Source: CAD feature listing. Evaluate the final solid. Frame: model axes, mm. Round coordinates to 2 decimals unless told otherwise and drop trailing zeros. Write each loop counter-clockwise with the first axis right and the second up, starting at its lowest first coordinate (ties: lowest second). Pieces come first, ordered by that corner, then holes. Notation, with made-up numbers: M 85.5,-3 L 130.5,-3 A22 ccw 130.5,24 Z; hole C 62.25,16 d11. An arc over 180 degrees is marked long. Answer in a Markdown table with one row per item.
from build123d import *

# Parameters (mm, degrees)
F1_DEPTH = 19.05
F2_R     = 76.2
F3_W     = 88.9
F3_H     = 38.1
F4_DEPTH = 38.1
F6_DEPTH = 38.101


with BuildPart() as f1:
    # F0 (on Front) → F1 (new body, symmetric)
    with BuildSketch(Plane.XZ):
        Polygon((-44.45, 0), (-19.05, 0), (19.05, 0), (44.45, 0), (330.2, -433.689813), (381, -433.689813), (117.024645, 76.2), (381, 290.210187), (292.1, 290.210187), (44.45, 152.4), (0, 152.4), (-44.45, 152.4), (-292.1, 290.210187), (-381, 290.210187), (-117.024645, 76.2), (-381, -433.689813), (-330.2, -433.689813), align=None)
    extrude(amount=F1_DEPTH, both=True)

    # F2
    f2_edges = [f1.edges().sort_by_distance(p)[0] for p in [
        (117.024645, 0, 76.2),
        (-44.45, 0, 152.4),
        (44.45, 0, 152.4),
        (-117.024645, 0, 76.2),
        (-44.45, 0, 0),
        (44.45, 0, 0),
    ]]
    fillet(f2_edges, radius=F2_R)

    # F3 (on face) → F4 (join)
    with BuildSketch(Plane.XY.offset(290.210187)):
        with Locations((-336.55, 0)):
            Rectangle(F3_W, F3_H)
        with Locations((336.55, 0)):
            Rectangle(F3_W, F3_H)
    extrude(amount=F4_DEPTH)

    # F5 (on face) → F6 (cut, through all)
    with BuildSketch(Plane.XZ.offset(19.05)):
        with BuildLine():
            Line((-19.05, 76.2), (-19.05, -1.623687))
            ThreePointArc((-19.05, -1.623687), (-11.268752, -0.407009), (-3.403482, 0))
            Line((-3.403482, 0), (3.403482, 0))
            ThreePointArc((3.403482, 0), (11.268752, -0.407009), (19.05, -1.623687))
            Line((19.05, -1.623687), (19.05, 76.2))
            Line((19.05, 76.2), (-19.05, 76.2))
        make_face()
        with BuildLine():
            Line((-19.05, -1.623687), (-19.05, -12.7))
            Line((-19.05, -12.7), (19.05, -12.7))
            Line((19.05, -12.7), (19.05, -1.623687))
            ThreePointArc((19.05, -1.623687), (11.268752, -0.407009), (3.403482, 0))
            Line((3.403482, 0), (-3.403482, 0))
            ThreePointArc((-3.403482, 0), (-11.268752, -0.407009), (-19.05, -1.623687))
        make_face()
    extrude(amount=-F6_DEPTH, mode=Mode.SUBTRACT)


solid = f1.part
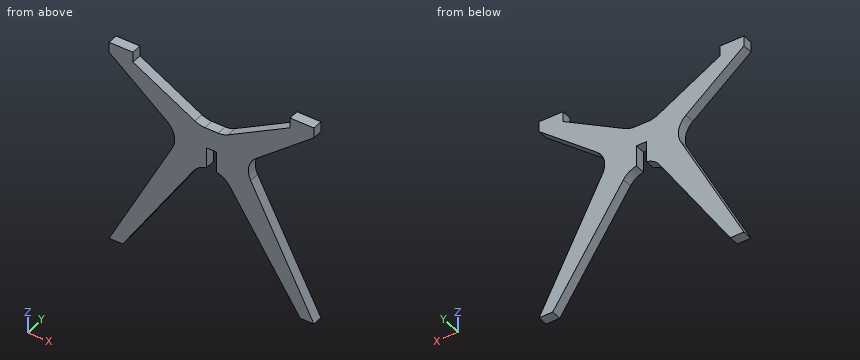
Q1. Contact query for flat-ended pins moving along their axis: pin 1 Ø19 at (y, z) = (9.5, 46) entering from +X; pin 2 Ø3 at (x, y) = (20.5, -11) entering from +Z; pin 3 Ø3 at (x, y) = (-133, 7) entering from +Z. Output: stop coordinate, or through.
Solutions:
| item | result |
|---|---|
| pin 1 | stops at x = 139.6 |
| pin 2 | stops at z = 152.4 |
| pin 3 | stops at z = 202.51 |
Q2. Section D-D (x = -86.5). Return loops of the section in (y, z).
Solutions:
| item | result |
|---|---|
| outline | M -19.05,-63.82 L 19.05,-63.82 L 19.05,175.8 L -19.05,175.8 Z |
Q3. Section C-C (x = 206.5). Return loops of the section in (y, z).
Solutions:
| item | result |
|---|---|
| outline | M -19.05,-245.95 L 19.05,-245.95 L 19.05,-96.63 L -19.05,-96.63 Z; M -19.05,148.74 L 19.05,148.74 L 19.05,242.58 L -19.05,242.58 Z |
Q4. Section A-A (z = 266). Return loops of the section in (x, y).
Solutions:
| item | result |
|---|---|
| outline | M -351.14,-19.05 L -248.59,-19.05 L -248.59,19.05 L -351.14,19.05 Z; M 248.59,-19.05 L 351.14,-19.05 L 351.14,19.05 L 248.59,19.05 Z |
Q5. Material intervals for probe 1 along X at (y, z) = (6, 56); probe 2 along Z at (x, y) = (261, 7); probe 3 along X at (y, z) = (-7.5, -11.5), sorted ascending.
Solutions:
| item | result |
|---|---|
| probe 1 | x = -137.04 to -19.05, 19.05 to 137.04 |
| probe 2 | z = -328.66 to -201.9, 192.92 to 272.9 |
| probe 3 | x = -162.43 to -43.66, 43.66 to 162.43 |
Q6. Section B-B (y = -2). Return loops of the section in (x, z).
Solutions:
| item | result |
|---|---|
| outline | M -381,-433.69 L -330.2,-433.69 L -67.03,-34.28 A76.2 cw -19.05,-1.62 L -19.05,76.2 L 19.05,76.2 L 19.05,-1.62 A76.2 cw 67.03,-34.28 L 330.2,-433.69 L 381,-433.69 L 145.57,21.07 A76.2 cw 165.25,115.3 L 381,290.21 L 381,328.31 L 292.1,328.31 L 292.1,290.21 L 61.73,162.02 A76.2 cw 24.68,152.4 L -24.68,152.4 A76.2 cw -61.73,162.02 L -292.1,290.21 L -292.1,328.31 L -381,328.31 L -381,290.21 L -165.25,115.3 A76.2 cw -145.57,21.07 Z |
